Part print with two shaded views. Sizes in mm from the minimum x, y, z corner. Round coordinates to 2 decimals unless told otherwise and drop trailing zeros. Loops run counter-clockwise (first coordinate to the right, second up) from the corner with the lowest first, then second, coordinate; pieces in that order, holes last. Notation, with made-up numbers: (-18.5, -31) -> (31.5, -31) arc R38 cw to (31.5, 7) -> close; hole circle Ø6 at (59.25, -9). An arc over 180 degrees is marked (long way). Use a Markdown table: item, result. Add a question column.
Item 1: Flat gauge pin, fed straight in: pin 1 (1 mm diameter, centred on x = 1.5, y = 5.5, fed in from -Z). Where does the tip first touch, or does it go through?
Item 2: Cut at B-B, the plane x = 2.8. List the corners of the cut face in (y, z).
Item 3: Cut at D-D, the plane z = 13.25. List the corners of the cut face in (x, y), plus the area to 3 significant figures.
Item 4: Cut at C-C, the plane z = 2. List the corners of the cut face in (x, y).
Item 5: Two-plate mould, pull along Z, no slides. Class the marked faces 1, 2 and 3: pulls with the +Z half, pulls with the -Z half, needs draft (parallel to the pull), parting line crosses it, or undercut.
Item 6: Cut at A-A, the plane y = 2.6. List the corners of the cut face in (x, z), plus the area to 3 significant figures.
Item 7: Probe line 1 (Y direction, x = 2.05, z = 3); line 2 (Z direction, x = 1.1, y = 3.3); line 3 (Y direction, x = 0.8, z = 3.5). List the from-to ranges inside material, lowest first. Write a range as [from, to].
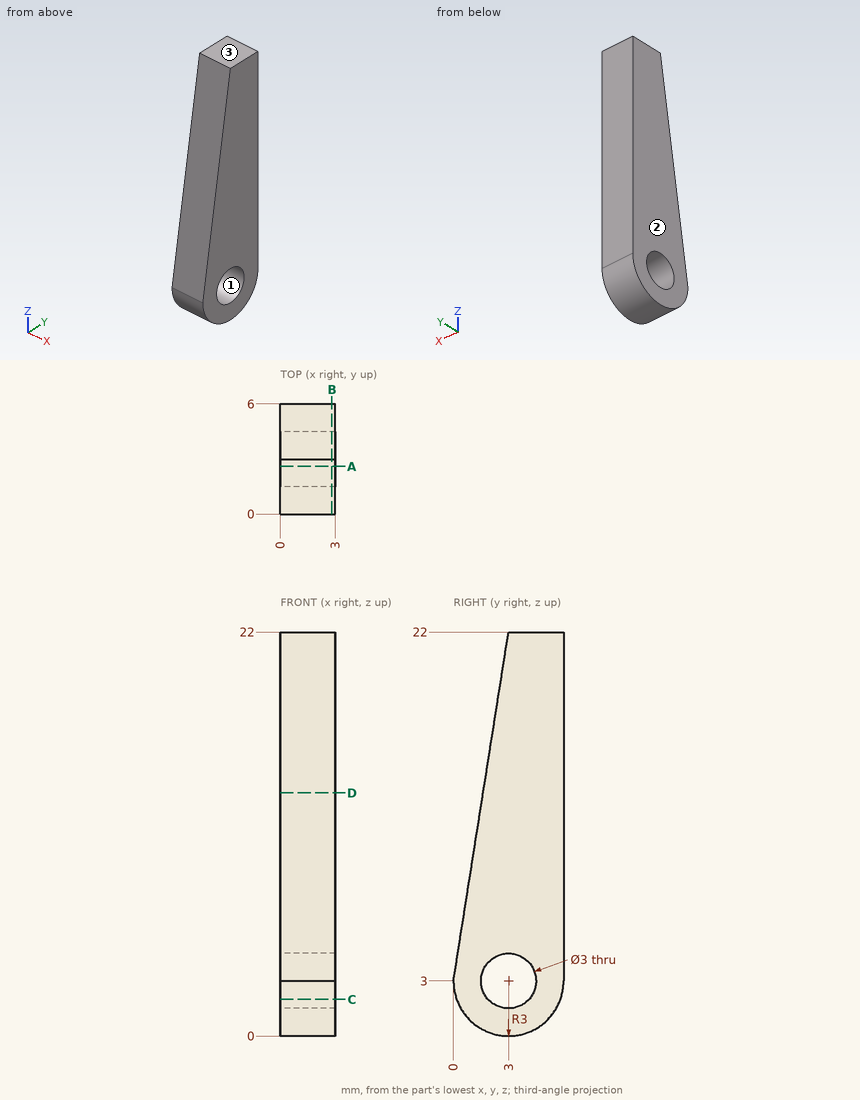
A:
| question | item | result |
|---|---|---|
| 1 | pin 1 | stops at z = 0.76 |
| 2 | outline | (0, 3) arc R3 ccw to (6, 3) -> (6, 22) -> (3, 22) -> close; hole circle Ø3 at (3, 3) |
| 3 | outline | (0, 1.62) -> (3, 1.62) -> (3, 6) -> (0, 6) -> close |
| 3 | area | 13.1 mm^2 |
| 4 | outline | (0, 0.17) -> (3, 0.17) -> (3, 1.88) -> (0, 1.88) -> close; (0, 4.12) -> (3, 4.12) -> (3, 5.83) -> (0, 5.83) -> close |
| 5 | face 1 | undercut |
| 5 | face 2 | needs draft |
| 5 | face 3 | pulls with the +Z half |
| 6 | outline | (0, 0.03) -> (3, 0.03) -> (3, 1.55) -> (0, 1.55) -> close; (0, 4.45) -> (3, 4.45) -> (3, 19.47) -> (0, 19.47) -> close |
| 6 | area | 49.6 mm^2 |
| 7 | line 1 | y = [0, 1.5], [4.5, 6] |
| 7 | line 2 | z = [0.02, 1.53], [4.47, 22] |
| 7 | line 3 | y = [0.08, 1.59], [4.41, 6] |
